from build123d import *
from OCP.BRepAlgoAPI import BRepAlgoAPI_Cut
from OCP.TopTools import TopTools_ListOfShape

# Parameters (mm, degrees)
BOSS_EXTRUDE1_DEPTH      = 11.938
BOSS_EXTRUDE1_DEPTH_BACK = 18.12511
SKETCH1_W                = 6.216067572
SKETCH1_H                = 27.404994669
BOSS_EXTRUDE2_DEPTH      = 27.404995
CUT_EXTRUDE1_DEPTH       = 4.179688
SKETCH4_R                = 0.95
CUT_EXTRUDE2_DEPTH       = 6.604
SKETCH7_W                = 5.699381266
SKETCH7_H                = 30.253154106
CUT_EXTRUDE3_DEPTH       = 31.242
SKETCH8_R                = 1.5
CUT_EXTRUDE4_DEPTH       = 32.004
SKETCH9_W                = 0.5
SKETCH9_H                = 26.458343153
CUT_EXTRUDE5_DEPTH       = 20


with BuildPart() as part:
    # Sketch1 → Boss-Extrude1 (new, two sides: drawn at the far end of the back side and taken through both)
    with BuildSketch(Plane(origin=(0, 0, 0), x_dir=(1, 0, 0), z_dir=(0, 1, 0)).offset(-BOSS_EXTRUDE1_DEPTH_BACK)):
        with Locations((-0.12984965, -1.559314439)):
            Rectangle(SKETCH1_W, SKETCH1_H)
    extrude(amount=BOSS_EXTRUDE1_DEPTH + BOSS_EXTRUDE1_DEPTH_BACK)

    # Sketch2 → Boss-Extrude2 (add)
    with BuildSketch(Plane(origin=(0, 0, -12.143182896), x_dir=(-1, 0, 0), z_dir=(0, 0, -1))):
        Polygon((15.337816326, 5.142144986), (3.237883436, 12.128044498), (-2.978184136, 12.128044498), (-2.978184136, 11.938), (3.237883436, 11.938), (3.237883436, -18.125109608), (9.640760589, -7.035001064), (8.050552579, -6.116894042), (8.197675426, -5.862069796), (12.657832776, 1.863149344), (14.248040785, 0.945042321), (15.067883436, 2.365051446), (16.337883436, 4.564755971), align=None)
    extrude(amount=-BOSS_EXTRUDE2_DEPTH)

    # Sketch3 → Cut-Extrude1 (cut)
    with BuildSketch(Plane(origin=(-6.061068176, 10.498078028, 0), x_dir=(0.866025403784441, 0.49999999999999606, 0), z_dir=(-0.49999999999999606, 0.866025403784441, 0))):
        Polygon((-11.866644114, -1.559314438), (-11.866644114, -7.909314438), (3.259932939, -7.909314438), (8.643205368, -7.909314438), (8.643205368, 4.790685562), (3.259932939, 4.790685562), (-11.866644114, 4.790685562), align=None)
    extrude(amount=-CUT_EXTRUDE1_DEPTH, mode=Mode.SUBTRACT)

    # Sketch4 → Cut-Extrude2 (cut)
    with BuildSketch(Plane(origin=(-10.27681526, -5.933322057, 0), x_dir=(0, 0, 1), z_dir=(-0.8660254037844423, -0.49999999999999406, 0))):
        with Locations(Location((12.245811773, 10.122136351, 0), (0, 0, 270))):
            Circle(SKETCH4_R)
        with Locations(Location((-9.154188227, 10.122136351, 0), (0, 0, 270))):
            Circle(SKETCH4_R)
        with Locations(Location((-9.154188227, -12.077863649, 0), (0, 0, 270))):
            Circle(SKETCH4_R)
        with Locations(Location((12.245811773, -12.077863649, 0), (0, 0, 270))):
            Circle(SKETCH4_R)
    extrude(amount=-CUT_EXTRUDE2_DEPTH, mode=Mode.SUBTRACT)


with BuildPart() as cut_extrude3_tool:
    # Sketch7 → Cut-Extrude3 (new body)
    with BuildSketch(Plane(origin=(0, 0, -12.143182896), x_dir=(-1, 0, 0), z_dir=(0, 0, -1))):
        with Locations((-0.128493503, -2.998532555)):
            Rectangle(SKETCH7_W, SKETCH7_H)
    extrude(amount=-CUT_EXTRUDE3_DEPTH)


with BuildPart() as part_1:
    add(part.part)

    # Cut-Extrude3: cut by cut_extrude3_tool, with a tolerance
    cut_extrude3_stock = TopTools_ListOfShape()
    cut_extrude3_stock.Append(part_1.part.wrapped)
    cut_extrude3_tools = TopTools_ListOfShape()
    cut_extrude3_tools.Append(cut_extrude3_tool.part.wrapped)
    cut_extrude3_cut = BRepAlgoAPI_Cut()
    cut_extrude3_cut.SetArguments(cut_extrude3_stock)
    cut_extrude3_cut.SetTools(cut_extrude3_tools)
    cut_extrude3_cut.SetFuzzyValue(0.00001)
    cut_extrude3_cut.Build()
    add(Compound.cast(cut_extrude3_cut.Shape()).solids(), mode=Mode.REPLACE)

    # Sketch8 → Cut-Extrude4 (cut)
    with BuildSketch(Plane(origin=(0, 0, -12.143182896), x_dir=(-1, 0, 0), z_dir=(0, 0, -1))):
        with Locations((5.32419713, 3.241176343)):
            Circle(SKETCH8_R)
    extrude(amount=-CUT_EXTRUDE4_DEPTH, mode=Mode.SUBTRACT)

    # Sketch9 → Cut-Extrude5 (cut)
    with BuildSketch(Plane(origin=(-10.27681526, -5.933322057, 0), x_dir=(0, 0, 1), z_dir=(-0.8660254037844423, -0.49999999999999406, 0))):
        with Locations((-11.893182896, -1.107035226)):
            Rectangle(SKETCH9_W, SKETCH9_H)
        with Locations((15.011811773, -1.107035226)):
            Rectangle(SKETCH9_W, SKETCH9_H)
    extrude(amount=-CUT_EXTRUDE5_DEPTH, mode=Mode.SUBTRACT)


solid = part_1.part
Source: CAD feature listing. Evaluate the final solid. Frame: model axes, mm. A direction names the side the tool comes from. Coordinates: 2 decimals unless noted, no trailing zeros. Loops run counter-clockwise (first coordinate to the right, second up) from the corner with the lowest first, then second, coordinate; pieces in that order, holes last. Notation, with made-up numbers: (15.25, 0) - (41.25, 0) arc R20 ccw to (41.25, 23) - close; hole circle Ø9 at (69.25, 13.5). An arc over 180 degrees is marked (long way). Return JSON: item names as keys, results as strings.
Q1. Section C-C, the plane z = 2.5. Return loops of the section in (x, y) (3 decimals), plus the area to 3 significant figures.
Results:
{"outline": "(-12.658, 1.863) - (-8.051, -6.117) - (-9.641, -7.035) - (-3.238, -18.125) - (-2.721, -18.125) - (-2.721, 7.6) - close; hole circle Ø3 at (-5.324, 3.241)", "area": "129 mm2"}
Q2. Mould query, pull axis Z, two halves, no side actions, for faces 1 (the flat face through (-6, -2, 14.762)), 2 (the flat face through (-8, 7, -4.791)), 3 (the flat face through (-6.395, -12.658, 1.374)). Classes: released by +Z, released by -Z, zero draft, split by the parting line, or undercut.
Results:
{"face 1": "released by +Z", "face 2": "undercut", "face 3": "zero draft"}
Q3. Material intervals for line 1 along Z through (x, y) = (-12, 6.5); line 2 along Y through (x, z) = (-8.75, -9.5); line 3 along Y through (x, z) = (-11, 12.5), sorted ascending.
Results:
{"line 1": "-11.64 to -4.79, 7.91 to 14.76", "line 2": "-8.58 to -6.52, -4.91 to 8.95", "line 3": "-1.01 to 4.28, 6.39 to 7.65"}
Q4. Section B-B, the plane y = 9. Return loops of the section in (x, z), plus the area to 3 significant figures.
Results:
{"outline": "(-8.66, -11.64) - (-2.72, -11.64) - (-2.72, -4.79) - (-8.66, -4.79) - close; (-8.66, 7.91) - (-2.72, 7.91) - (-2.72, 14.76) - (-8.66, 14.76) - close", "area": "81.3 mm2"}
Q5. Section A-A, the plane x = -5.25. Return loops of the section in (y, z), plus the area to 3 significant figures.
Results:
{"outline": "(-14.64, -11.64) - (1.74, -11.64) - (1.74, 14.76) - (-14.64, 14.76) - close; (4.74, -11.64) - (10.97, -11.64) - (10.97, -4.79) - (6.14, -4.79) - (6.14, 7.91) - (10.97, 7.91) - (10.97, 14.76) - (4.74, 14.76) - close", "area": "536 mm2"}
Q6. Access query for faces 4 (the flat face through (-13.44, 1.41, 11.29)), 5 (the flat face through (-8.857, -6.582, 1.374)), 6 (the flat face through (-9.6, 6.1, -9.1)). Directions: +Z, -Z, +X, -X, +Y, -Y. A direction counts if a zero-diameter tool reaches every point of the face in a straight line with its end or side. Return the directions, or none.
Results:
{"face 4": "+Z, -Z, -Y", "face 5": "+Z, -Z, -X", "face 6": "none"}
Q7. Section D-D, the plane x = -13.5. Give the number of separate pieces and of enclosed holes in the cut face, plus the area to 3 significant figures.
Results:
{"separate pieces": "2", "enclosed holes": "2", "area": "59.6 mm2"}
Q8. Contact query for flat-ended pins moving along their axis: P1, Ø3, axis at y = -8, z = -4.5, coming from the -X side; P2, Ø1.5, axis at x = -9.5, z = 5.5, coming from the -Y side; P3, Ø4, axis at x = -8.5, z = -7.5, coming from the +Y side. Output: stop coordinate, or through.
Results:
{"P1": "x = -9.64", "P2": "y = -8.58", "P3": "y = 10.24"}
